Input: part model. Units: mm. Frame: model coordinates. Round coordinates to 2 decimals unless told otherwise and drop trailing zeros. Loops run counter-clockwise (first coordinate to the right, second up) from the corner with the lowest first, then second, coordinate; pieces in that order, holes last.
1) Draft query along Y for faces 1 (the face through (-1, 0, 0)), 2 (the face through (-24, -23, 1.6)). Return one class per face: pulls with the +Y half, pulls with the -Y half, needs draft (parallel to the pull), parting line crosses it, or undercut.
2) Ray query, line 1 along Z through (x, y) = (31, 4). Return the intervals inside material, ascending.
3) First-contact query: pin 1 (1.2 mm diameter, centred on x = -58, y = -18.5, fed in from +Z). Flat tip, straight axial feed; report the tip coordinate or a pass-through.
4) Section A-A, the plane x = -52.5. Return loops of the section in (y, z).
from build123d import *

# Parameters (mm, degrees)
SKETCH1_W           = 122
SKETCH1_H           = 60
BOSS_EXTRUDE1_DEPTH = 1.5
SKETCH2_R           = 0.75
BOSS_EXTRUDE2_DEPTH = 0.01
SKETCH3_W           = 13
SKETCH3_H           = 13
BOSS_EXTRUDE3_DEPTH = 0.1
SKETCH4_W           = 13
SKETCH4_H           = 13
SKETCH4_W_2         = 12.6
SKETCH4_H_2         = 12.6
BOSS_EXTRUDE4_DEPTH = 0.1


with BuildPart() as part:
    # Sketch1 → Boss-Extrude1 (new body)
    with BuildSketch(Plane.XY):
        Rectangle(SKETCH1_W, SKETCH1_H)
    extrude(amount=BOSS_EXTRUDE1_DEPTH)

    # Sketch2 → Boss-Extrude2 (add)
    with BuildSketch(Plane.XY.offset(1.5)):
        with Locations(Location((60, -2, 0), (0, 0, 180))):
            Circle(SKETCH2_R)
        with Locations(Location((57.46, -2, 0), (0, 0, 180))):
            Circle(SKETCH2_R)
        with Locations(Location((54.92, -2, 0), (0, 0, 180))):
            Circle(SKETCH2_R)
        with Locations(Location((52.38, -2, 0), (0, 0, 180))):
            Circle(SKETCH2_R)
        with Locations(Location((49.84, -2, 0), (0, 0, 180))):
            Circle(SKETCH2_R)
        with Locations(Location((47.3, -2, 0), (0, 0, 180))):
            Circle(SKETCH2_R)
        with Locations(Location((44.76, -2, 0), (0, 0, 180))):
            Circle(SKETCH2_R)
        with Locations(Location((42.22, -2, 0), (0, 0, 180))):
            Circle(SKETCH2_R)
        with Locations(Location((57.46, -19.5, 0), (0, 0, 180))):
            Circle(SKETCH2_R)
        with Locations(Location((54.92, -19.5, 0), (0, 0, 180))):
            Circle(SKETCH2_R)
        with Locations(Location((52.38, -19.5, 0), (0, 0, 180))):
            Circle(SKETCH2_R)
        with Locations(Location((49.84, -19.5, 0), (0, 0, 180))):
            Circle(SKETCH2_R)
        with Locations(Location((47.3, -19.5, 0), (0, 0, 180))):
            Circle(SKETCH2_R)
        with Locations(Location((44.76, -19.5, 0), (0, 0, 180))):
            Circle(SKETCH2_R)
        with Locations(Location((42.22, -19.5, 0), (0, 0, 180))):
            Circle(SKETCH2_R)
        with Locations(Location((60, -19.5, 0), (0, 0, 180))):
            Circle(SKETCH2_R)
        with Locations(Location((39.68, -2, 0), (0, 0, 180))):
            Circle(SKETCH2_R)
        with Locations(Location((39.68, -4.5, 0), (0, 0, 180))):
            Circle(SKETCH2_R)
        with Locations(Location((39.68, -7, 0), (0, 0, 180))):
            Circle(SKETCH2_R)
        with Locations(Location((39.68, -9.5, 0), (0, 0, 180))):
            Circle(SKETCH2_R)
        with Locations(Location((39.68, -12, 0), (0, 0, 180))):
            Circle(SKETCH2_R)
        with Locations(Location((39.68, -14.5, 0), (0, 0, 180))):
            Circle(SKETCH2_R)
        with Locations(Location((39.68, -17, 0), (0, 0, 180))):
            Circle(SKETCH2_R)
        with Locations(Location((39.68, -19.5, 0), (0, 0, 180))):
            Circle(SKETCH2_R)
        with Locations(Location((55, 24, 0), (0, 0, 180))):
            Circle(SKETCH2_R)
        with Locations(Location((22.5, 24, 0), (0, 0, 180))):
            Circle(SKETCH2_R)
        with Locations(Location((22.5, 21.46, 0), (0, 0, 180))):
            Circle(SKETCH2_R)
        with Locations(Location((22.5, 18.92, 0), (0, 0, 180))):
            Circle(SKETCH2_R)
        with Locations(Location((22.5, 16.38, 0), (0, 0, 180))):
            Circle(SKETCH2_R)
        with Locations(Location((22.5, 13.84, 0), (0, 0, 180))):
            Circle(SKETCH2_R)
        with Locations(Location((22.5, 11.3, 0), (0, 0, 180))):
            Circle(SKETCH2_R)
        with Locations(Location((22.5, 8.76, 0), (0, 0, 180))):
            Circle(SKETCH2_R)
        with Locations(Location((22.5, 6.22, 0), (0, 0, 180))):
            Circle(SKETCH2_R)
        with Locations(Location((55, 21.46, 0), (0, 0, 180))):
            Circle(SKETCH2_R)
        with Locations(Location((55, 18.92, 0), (0, 0, 180))):
            Circle(SKETCH2_R)
        with Locations(Location((55, 16.38, 0), (0, 0, 180))):
            Circle(SKETCH2_R)
        with Locations(Location((55, 13.84, 0), (0, 0, 180))):
            Circle(SKETCH2_R)
        with Locations(Location((55, 11.3, 0), (0, 0, 180))):
            Circle(SKETCH2_R)
        with Locations(Location((55, 8.76, 0), (0, 0, 180))):
            Circle(SKETCH2_R)
        with Locations(Location((55, 6.22, 0), (0, 0, 180))):
            Circle(SKETCH2_R)
        with Locations(Location((10, 25, 0), (0, 0, 180))):
            Circle(SKETCH2_R)
        with Locations(Location((7.46, 25, 0), (0, 0, 180))):
            Circle(SKETCH2_R)
        with Locations(Location((4.92, 25, 0), (0, 0, 180))):
            Circle(SKETCH2_R)
        with Locations(Location((2.38, 25, 0), (0, 0, 180))):
            Circle(SKETCH2_R)
        with Locations(Location((-0.16, 25, 0), (0, 0, 180))):
            Circle(SKETCH2_R)
        with Locations(Location((-2.7, 25, 0), (0, 0, 180))):
            Circle(SKETCH2_R)
        with Locations(Location((-58, -21, 0), (0, 0, 180))):
            Circle(SKETCH2_R)
        with Locations(Location((-58, -18.46, 0), (0, 0, 180))):
            Circle(SKETCH2_R)
        with Locations(Location((-58, -15.92, 0), (0, 0, 180))):
            Circle(SKETCH2_R)
        with Locations(Location((-58, -13.38, 0), (0, 0, 180))):
            Circle(SKETCH2_R)
        with Locations(Location((-58, -10.84, 0), (0, 0, 180))):
            Circle(SKETCH2_R)
        with Locations(Location((-58, -8.3, 0), (0, 0, 180))):
            Circle(SKETCH2_R)
        with Locations(Location((20, -1, 0), (0, 0, 180))):
            Circle(SKETCH2_R)
        with Locations(Location((22.54, -1, 0), (0, 0, 180))):
            Circle(SKETCH2_R)
        with Locations(Location((22.54, -3.54, 0), (0, 0, 180))):
            Circle(SKETCH2_R)
        with Locations(Location((22.54, -6.08, 0), (0, 0, 180))):
            Circle(SKETCH2_R)
        with Locations(Location((22.54, -8.62, 0), (0, 0, 180))):
            Circle(SKETCH2_R)
        with Locations(Location((20, -3.54, 0), (0, 0, 180))):
            Circle(SKETCH2_R)
        with Locations(Location((20, -6.08, 0), (0, 0, 180))):
            Circle(SKETCH2_R)
        with Locations(Location((20, -8.62, 0), (0, 0, 180))):
            Circle(SKETCH2_R)
        with Locations(Location((29, -1, 0), (0, 0, 180))):
            Circle(SKETCH2_R)
        with Locations(Location((31.54, -1, 0), (0, 0, 180))):
            Circle(SKETCH2_R)
        with Locations(Location((31.54, -3.54, 0), (0, 0, 180))):
            Circle(SKETCH2_R)
        with Locations(Location((29, -3.54, 0), (0, 0, 180))):
            Circle(SKETCH2_R)
        with Locations(Location((29, -6.08, 0), (0, 0, 180))):
            Circle(SKETCH2_R)
        with Locations(Location((29, -8.62, 0), (0, 0, 180))):
            Circle(SKETCH2_R)
        with Locations(Location((31.54, -8.62, 0), (0, 0, 180))):
            Circle(SKETCH2_R)
        with Locations(Location((31.54, -6.08, 0), (0, 0, 180))):
            Circle(SKETCH2_R)
        with Locations(Location((23, -16, 0), (0, 0, 180))):
            Circle(SKETCH2_R)
        with Locations(Location((20.46, -16, 0), (0, 0, 180))):
            Circle(SKETCH2_R)
        with Locations(Location((17.92, -16, 0), (0, 0, 180))):
            Circle(SKETCH2_R)
        with Locations(Location((15.38, -16, 0), (0, 0, 180))):
            Circle(SKETCH2_R)
        with Locations(Location((20.46, -18.54, 0), (0, 0, 180))):
            Circle(SKETCH2_R)
        with Locations(Location((17.92, -18.54, 0), (0, 0, 180))):
            Circle(SKETCH2_R)
        with Locations(Location((15.38, -18.54, 0), (0, 0, 180))):
            Circle(SKETCH2_R)
        with Locations(Location((23, -18.54, 0), (0, 0, 180))):
            Circle(SKETCH2_R)
    extrude(amount=BOSS_EXTRUDE2_DEPTH)

    # Sketch3 → Boss-Extrude3 (add)
    with BuildSketch(Plane.XY.offset(1.5)):
        with Locations((-24, -23.5)):
            Rectangle(SKETCH3_W, SKETCH3_H)
    extrude(amount=BOSS_EXTRUDE3_DEPTH)

    # Sketch4 → Boss-Extrude4 (add)
    with BuildSketch(Plane.XY.offset(1.6)):
        with Locations((-24, -23.5)):
            Rectangle(SKETCH4_W, SKETCH4_H)
        with Locations((-24, -23.5)):
            Rectangle(SKETCH4_W_2, SKETCH4_H_2, mode=Mode.SUBTRACT)
    extrude(amount=BOSS_EXTRUDE4_DEPTH)


solid = part.part
Final values:
1. face 1: needs draft
1. face 2: undercut
2. line 1: z = 0 to 1.5
3. pin 1: stops at z = 1.51
4. outline: (-30, 0) - (30, 0) - (30, 1.5) - (-30, 1.5) - close
